```python
from build123d import *

# Parameters (mm, degrees)
F0_W     = 12.5
F0_H     = 48
F1_DEPTH = 3.5
F2_W     = 5.2
F2_H     = 8.2
F3_DEPTH = 2.2
F4_W     = 2
F4_H     = 5.4
F5_DEPTH = 3.5
F6_R     = 2
F7_DEPTH = 2.2


# Not quite as in the source:
# - a feature names something its author has since deleted; it is built from what else it names


with BuildPart() as f1:
    # F0 (on Front) → F1 (new body)
    with BuildSketch(Plane.XZ):
        Rectangle(F0_W, F0_H)
    extrude(amount=-F1_DEPTH)

    # F2 (on Front) → F3 (cut)
    with BuildSketch(Plane.XZ):
        with Locations((0, -15.5)):
            Rectangle(F2_W, F2_H)
    extrude(amount=-F3_DEPTH, mode=Mode.SUBTRACT)

    # F4 (on Front) → F5 (cut)
    with BuildSketch(Plane.XZ):
        with Locations((0, -15.5)):
            Rectangle(F4_W, F4_H)
    extrude(amount=-F5_DEPTH, mode=Mode.SUBTRACT)

    # F6 (on Front) → F7 (cut)
    with BuildSketch(Plane.XZ):
        with Locations((0, -11.4)):
            Circle(F6_R)
    extrude(amount=-F7_DEPTH, mode=Mode.SUBTRACT)


solid = f1.part
```
Read the model definition and answer for the solid it produces. Units are mm, in the model's axes. A direction names the side the tool comes from. Coordinates: 2 decimals unless noted, no trailing zeros. Order: outer loops, then holes, each group sorted by start corner. A loop starts at its lowest first (then second) coordinate and runs counter-clockwise, first axis right, second up. Notation, with made-up numbers: (38.5, 83) - (84.5, 83) arc R13 ccw to (84.5, 100) - close; hole circle Ø5 at (0.25, -26). An arc over 180 degrees is marked (long way). Answer as a JSON object with one key per item and string values. Group by question number.
Item 1: Section B-B (y = 1.3) is taken. Give the vertices of the cut face in (x, z), plus the area to 3 significant figures.
Item 2: A tool of negligible diameter and unlimited length cuts with its end or side. For faces 1 (the face through (-2.6, 1, -16)), 2 (the face through (-6.25, 2, 0)), 3 (the face through (1, 3, -16)), from which of +Z, -Z, +X, -X, +Y, -Y can it reach the whole face along a straight path? Write none if from no direction.
Item 3: Consider probe 1 along X at (y, z) = (1.5, -12.5); probe 2 along Z at (x, y) = (-2.25, 1.2); probe 3 along Z at (x, y) = (-0.5, 2.7). Determine where each line is inside the solid, lowest interval first. Write a range as from..to.
Item 4: Section A-A (x = 0) is taken. Give the vertices of the cut face in (y, z), plus the area to 3 significant figures.
Item 5: The mould has two halves that part along X. Classify faces 4 (the face through (0, 2, -24)), 5 (the face through (0, 1, -19.6)), 6 (the face through (6.25, 2, 0)): +X half, -X half, draft (parallel to the pull), parting line (faces both ways), or undercut.
Item 6: A flat-ended cylindrical pin translates along its axis: P1, Ø4, axis at x = 0.5, z = -15, coming from the -Y side. Find the tip coordinate at first contact, or state that the pin passes through.
Results are:
{
 "1": {"outline": "(-6.25, -24) - (6.25, -24) - (6.25, 24) - (-6.25, 24) - close; hole (-2.6, -19.6) - (2.6, -19.6) - (2.6, -11.4) - (2, -11.4) arc R2 ccw to (-2, -11.4) - (-2.6, -11.4) - close", "area": "551 mm^2"},
 "2": {"face 1": "-Y", "face 2": "+Z, -Z, -X, +Y, -Y", "face 3": "+Y, -Y"},
 "3": {"probe 1": "x = -6.25..-2.6, 2.6..6.25", "probe 2": "z = -24..-19.6, -11.4..24", "probe 3": "z = -24..-18.2, -12.8..24"},
 "4": {"outline": "(0, -24) - (3.5, -24) - (3.5, -18.2) - (2.2, -18.2) - (2.2, -19.6) - (0, -19.6) - close; (0, -9.4) - (2.2, -9.4) - (2.2, -12.8) - (3.5, -12.8) - (3.5, 24) - (0, 24) - close", "area": "139 mm^2"},
 "5": {"face 4": "draft", "face 5": "undercut", "face 6": "+X half"},
 "6": {"P1": "stops at y = 2.2"}
}
